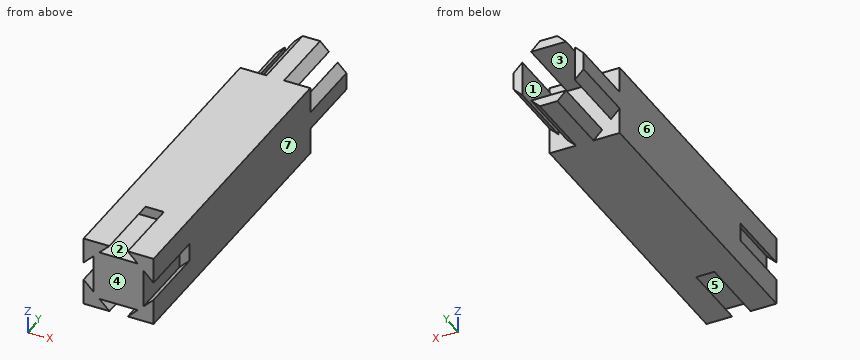
Autodesk Inventor part; units mm, degrees
ref_plane "YZ Plane" through (0, 0, 0) normal (1, 0, 0) x (0, 1, 0)
ref_plane "XZ Plane" through (0, 0, 0) normal (0, 1, 0) x (-1, 0, 0)
ref_plane "XY Plane" through (0, 0, 0) normal (0, 0, 1) x (1, 0, 0)
sketch "Skizze1" plane through (0, 0, 0) normal (0, 1, 0) x (-1, 0, 0)
  line L0 (15, 15) -> (-15, 15)
  line L1 (-15, 15) -> (-15, -15)
  line L2 (-15, -15) -> (15, -15)
  line L3 (15, -15) -> (15, 15)
  line L4 (15, 0) -> (11, 0) construction
  line L5 (11.25, 7.5042) -> (11.25, -7.4958)
  line L6 (15, 3.75) -> (15, -3.75)
  line L7 (11.25, 7.5042) -> (15, 3.75)
  line L8 (11.25, -7.4958) -> (15, -3.75)
  line L9 (-7.5042, 11.25) -> (-3.75, 15)
  line L10 (-7.5042, 11.25) -> (7.4958, 11.25)
  line L11 (7.4958, 11.25) -> (3.75, 15)
  line L12 (15, 15) -> (-15, 15)
  line L13 (-11.25, -7.5042) -> (-15, -3.75)
  line L14 (-11.25, -7.5042) -> (-11.25, 7.4958)
  line L15 (-11.25, 7.4958) -> (-15, 3.75)
  line L16 (-15, 15) -> (-15, -15)
  line L17 (7.5042, -11.25) -> (3.75, -15)
  line L18 (7.5042, -11.25) -> (-7.4958, -11.25)
  line L19 (-7.4958, -11.25) -> (-3.75, -15)
  line L20 (-15, -15) -> (15, -15)
  line L21 (15, -15) -> (-15, -15)
  line L22 (-15, -15) -> (-15, 15)
  line L23 (-15, 15) -> (15, 15)
  line L24 (15, 15) -> (15, -15)
  point P0 (0, 0)
  point P1 (0, 15)
  point P2 (-15, 0)
  point P3 (0, -15)
  point P4 (-3.75, -15)
  point P5 (3.75, -15)
  point P6 (-15, 3.75)
  point P7 (-15, -3.75)
  point P8 (3.75, 15)
  point P9 (-3.75, 15)
  dimension "d0" = 15
  dimension "d1" = 30
  dimension "d2" = 30
  dimension "d3" = 15
  dimension "d4" = 4
  dimension "d5" = 15
  dimension "d6" = 7.5
  dimension "d7" = 7.5
  dimension "d8" = 3.75
  dimension "d11" = 360
extrude "Extrusion1" add sketch "Skizze1" along normal blind 30 contours L11 L10 L9 L0 | L3 L8 L5 L7 | L15 L14 L13 L1 | L2 L19 L18 L17
extrude "Extrusion2" add sketch "Skizze1" against normal blind 70
sketch "Skizze4" plane through (0, -70, 0) normal (0, -1, 0) x (1, 0, 0)
  line L0 (-15.2121, -3.7121) -> (-10.7, -8.2243)
  line L1 (-10.7, -8.2243) -> (-10.7, 8.2243)
  line L2 (-10.7, 8.2243) -> (-15.2121, 3.7121)
  line L3 (-15, -3.9243) -> (-15, 3.9243)
  line L4 (3.7121, -15.2121) -> (8.2243, -10.7)
  line L5 (8.2243, -10.7) -> (-8.2243, -10.7)
  line L6 (-8.2243, -10.7) -> (-3.7121, -15.2121)
  line L7 (3.9243, -15) -> (-3.9243, -15)
  line L8 (15.2121, 3.7121) -> (10.7, 8.2243)
  line L9 (10.7, 8.2243) -> (10.7, -8.2243)
  line L10 (10.7, -8.2243) -> (15.2121, -3.7121)
  line L11 (15, 3.9243) -> (15, -3.9243)
  line L12 (-3.7121, 15.2121) -> (-8.2243, 10.7)
  line L13 (-8.2243, 10.7) -> (8.2243, 10.7)
  line L14 (8.2243, 10.7) -> (3.7121, 15.2121)
  line L15 (-3.9243, 15) -> (3.9243, 15)
  line L16 (-15, 15) -> (-3.75, 15)
  line L17 (-15, 15) -> (15, 15)
  line L18 (15, 15) -> (15, -15)
  line L19 (15, -15) -> (-15, -15)
  line L20 (-15, -15) -> (-15, 15)
  point P0 (0, 0)
  point P1 (0, 0)
  point P2 (-290.3305, 55.2757)
  point P3 (-298.179, 55.2757)
  point P4 (-3.9243, 15)
  dimension "d27" = 360
extrude "Extrusion4" add sketch "Skizze4" along normal blind 30
sketch "Skizze5" plane through (0, -100, 0) normal (0, -1, 0) x (1, 0, 0)
  line L0 (18.5438, 0) -> (-21.4353, 0) construction
  line L1 (-11, 7.5) -> (-11, -7.5)
  line L2 (-11, 7.5) -> (-15, 3.5)
  line L3 (-11, -7.5) -> (-15, -3.5)
  line L4 (-15.2121, -3.7121) -> (-10.7, -8.2243)
  line L5 (-10.7, -8.2243) -> (-10.7, 8.2243)
  line L6 (-10.7, 8.2243) -> (-15.2121, 3.7121)
  line L7 (-15, -3.9243) -> (-15, 3.9243)
  line L8 (3.7121, -15.2121) -> (8.2243, -10.7)
  line L9 (8.2243, -10.7) -> (-8.2243, -10.7)
  line L10 (-8.2243, -10.7) -> (-3.7121, -15.2121)
  line L11 (3.9243, -15) -> (-3.9243, -15)
  line L12 (15.2121, 3.7121) -> (10.7, 8.2243)
  line L13 (10.7, 8.2243) -> (10.7, -8.2243)
  line L14 (10.7, -8.2243) -> (15.2121, -3.7121)
  line L15 (15, 3.9243) -> (15, -3.9243)
  line L16 (-3.7121, 15.2121) -> (-8.2243, 10.7)
  line L17 (-8.2243, 10.7) -> (8.2243, 10.7)
  line L18 (8.2243, 10.7) -> (3.7121, 15.2121)
  line L19 (-3.9243, 15) -> (3.9243, 15)
  line L20 (15, 15) -> (-15, 15)
  line L21 (3.9243, 15) -> (15, 15)
  line L22 (15, 15) -> (15, 3.9243)
  line L23 (15, -3.9243) -> (15, -15)
  line L24 (15, -15) -> (3.9243, -15)
  line L25 (-3.9243, -15) -> (-15, -15)
  line L26 (-15, -15) -> (-15, -3.9243)
  line L27 (-15, 3.9243) -> (-15, 15)
  line L28 (-15, 15) -> (-3.9243, 15)
  point P0 (0, 0)
  dimension "d34" = 15
  dimension "d38" = 0.3
  dimension "d39" = 360
extrude "Extrusion5" add sketch "Skizze5" along normal blind 30 contours L27 L20 L16 L17 L18 L22 L12 L13 L14 L23 L24 L8 L9 L10 L25 L26 L4 L5 L6
equation "\"d6\" = 0.5 * d5"
equation "\"d8\" = 0.5 * d7"
properties part number "TestEbene2"
For this review, take the finished solid that the model builds, in its own axes (mm). Face numbers are marked on the shaded views. A direction names the side the tool comes from. Give positions to 0.01 mm unless a question says otherwise; leave off trailing zeros. Order: outer loops, then holes, each group sorted by start corner. A loop starts at its lowest first (then second) coordinate and runs counter-clockwise, first axis right, second up.
1) Take a section at B-B (x = 2). Give the boundary of the cut face in (y, z).
2) Wall thickness on line 1 (Z direction, x = -5.25, y = -118.5); line 2 (Z direction, x = 6, y = -123); line 3 (Z direction, x = 0, y = -109): over which ranges is each line inside the solid? List them lowest first.
3) The part is to be moulded in two halves that separate along X. For the marked faces 5, 6 and 7, say which applies: released by +X, released by -X, zero draft, split by the parting line, or undercut.
4) Insertion check: pin 1 (18 mm diameter, centred on x = 0.5, y = -108, fed in from +Z); pin 2 (9 mm diameter, centred on x = 1.5, z = -1, fed in from +Y); pin 3 (3.5 mm diameter, centred on x = 1.5, z = -12.5, fed in from -Y). Each pin has a flat end and moves straight along its axis. Give the tip position at first contact, or say it passes through.
5) Take a section at A-A (z = 2). Give the boundary of the cut face in (x, y).
6) For the marked faces 1, 2, 3 and 4, list the 3-axis set-ups (+Z, -Z, +X, -X, +Y, -Y) from which the entire face can be reached by the end or side of a thin tool; tool diameter is ignored.
Derived:
1. outline: (-130, -10.7) - (-100, -10.7) - (-100, -15) - (30, -15) - (30, -11.25) - (0, -11.25) - (0, 11.25) - (30, 11.25) - (30, 15) - (-100, 15) - (-100, 10.7) - (-130, 10.7) - close
2. line 1: z = -15 to -13.67, -10.7 to 10.7, 13.67 to 15
2. line 2: z = -15 to -12.92, -10.7 to 10.7, 12.92 to 15
2. line 3: z = -10.7 to 10.7
3. face 5: undercut
3. face 6: released by -X
3. face 7: released by +X
4. pin 1: stops at z = 15
4. pin 2: stops at y = 0
4. pin 3: stops at y = -100
5. outline: (-15, -100) - (-10.7, -100) - (-10.7, -130) - (10.7, -130) - (10.7, -100) - (15, -100) - (15, 30) - (11.25, 30) - (11.25, 0) - (-11.25, 0) - (-11.25, 30) - (-15, 30) - close
6. face 1: +Z, -Z, +Y
6. face 2: -Y
6. face 3: +X, -X, +Y
6. face 4: +Z, -Z, +X, -X, -Y
